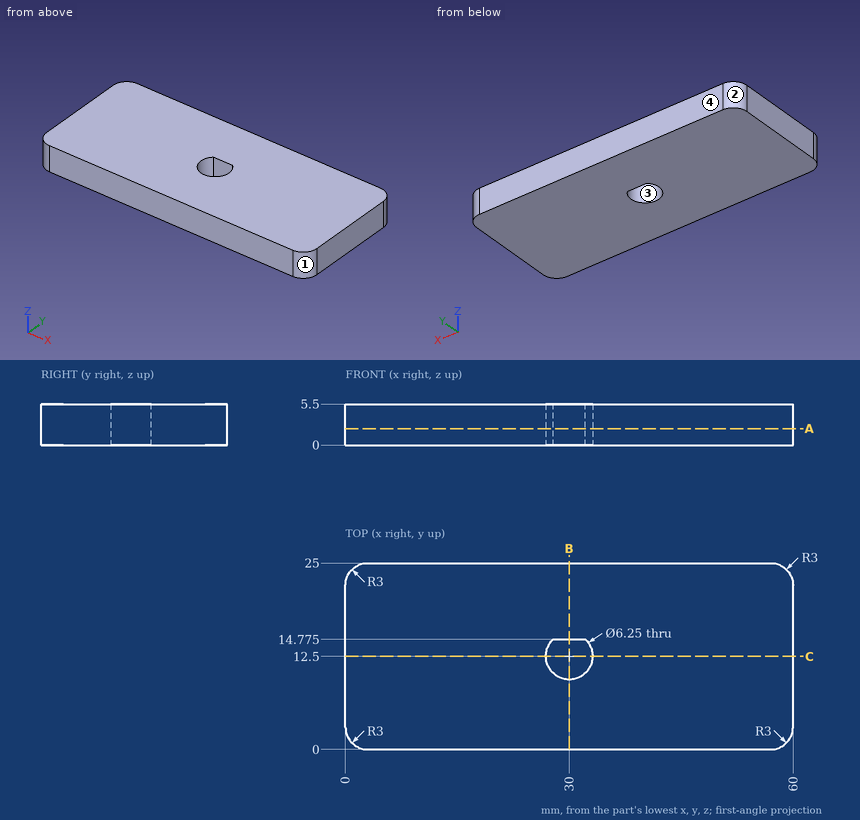
Study the drawing (mm; zero at the part's minimum x, y, z) and answer. Give positions to 0.01 mm unless a question says otherwise; leave off trailing zeros. Order: outer loops, then holes, each group sorted by start corner. A loop starts at its lowest first (then second) coordinate and runs counter-clockwise, first axis right, second up. Notation, with made-up numbers: (-8.5, -12) -> (33.5, -12) arc R38 cw to (33.5, 26) -> close; hole circle Ø2 at (43.5, -10). An arc over 180 degrees is marked (long way). Put each result on its own line as item: value.
Item 1: A cutting plane is placed at C-C on y = 12.5. Give the vertices of the cut face in (x, z) (3 decimals), plus the area to 3 significant figures.
Established:
outline: (0, 0) -> (26.875, 0) -> (26.875, 5.5) -> (0, 5.5) -> close; (33.125, 0) -> (60, 0) -> (60, 5.5) -> (33.125, 5.5) -> close
area: 296 mm^2
Item 2: Straight lines are drawn through the part: line 1 (Y direction, x = 30, z = 1.5) (3 decimals); line 2 (X direction, y = 12.5, z = 2.4) (3 decimals); line 3 (X direction, y = 11, z = 4.1). For each, find the intervals that lie inside material, in ascending order.
Established:
line 1: y = 0 to 9.375, 14.775 to 25
line 2: x = 0 to 26.875, 33.125 to 60
line 3: x = 0 to 27.26, 32.74 to 60
Item 3: A cutting plane is placed at A-A on z = 2.2. Give the vertices of the cut face in (x, y) (3 decimals).
Established:
outline: (0, 3) arc R3 ccw to (3, 0) -> (57, 0) arc R3 ccw to (60, 3) -> (60, 22) arc R3 ccw to (57, 25) -> (3, 25) arc R3 ccw to (0, 22) -> close; hole (27.858, 14.775) arc R3.125 ccw (long way) to (32.142, 14.775) -> close
Item 4: A cutting plane is placed at B-B on x = 30. Give the vertices of the cut face in (y, z) (3 decimals).
Established:
outline: (0, 0) -> (9.375, 0) -> (9.375, 5.5) -> (0, 5.5) -> close; (14.775, 0) -> (25, 0) -> (25, 5.5) -> (14.775, 5.5) -> close
Item 5: For a pull along X with two mould halves and no side action, classify the marked faces 1, 2, 3 and 4 as released by +X, released by -X, zero draft, split by the parting line, or undercut.
Established:
face 1: released by +X
face 2: released by -X
face 3: undercut
face 4: zero draft
